Part model, mm, in its own coordinate system. Face numbers are marked on the shaded views. A direction names the side the tool comes from. Coordinates: 2 decimals unless noted, no trailing zeros. Loops run counter-clockwise (first coordinate to the right, second up) from the corner with the lowest first, then second, coordinate; pieces in that order, holes last. Notation, with made-up numbers: (31.25, 63) - (82.25, 63) arc R16 cw to (82.25, 68) - close; hole circle Ø3 at (-31, 20). An arc over 180 degrees is marked (long way). Use a Markdown table: item, result. Add a question column.
1) Band-saw the part on B-B (x = 0). Give the cut face in (y, z).
2) Probe probe 1 along X at (y, z) = (-3.25, -3); probe 2 along Y at (x, z) = (-6.5, 7); probe 3 along X at (y, z) = (8.5, -2). List the from-to ranges inside material, lowest first. Write a range as [from, to].
3) Band-saw the part on A-A (z = 0). Give the cut face in (x, y).
4) Pull direction Z, two halves, no side cores. Call the marked faces 3, 4 and 5: +Z half, -Z half, draft (parallel to the pull), parting line (faces both ways), or undercut.
5) Band-saw the part on C-C (y = -2). Give the cut face in (x, z).
6) Band-saw the part on D-D (y = 13). Give the cut face in (x, z).
7) Drop flat-ended pins along their axis: P1, Ø3, axis at y = 3.5, z = 6.5, coming from the -X side; P2, Ø4, axis at x = 13.5, y = 0.5, coming from the -Z side; P3, Ø6, axis at x = 11.5, z = 9, coming from the -Y side. Give the stop position or say it passes through.
8) Tool access for the marked faces 1 and 2: list every direction of +Z, -Z, +X, -X, +Y, -Y with a clear straight run to the whole face (end or side of a thin tool).
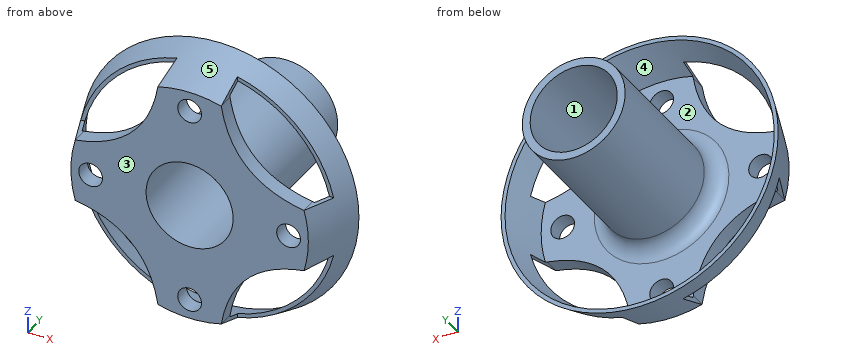
from build123d import *

# Parameters (mm, degrees)
SKETCH1_R           = 17.5
BOSS_EXTRUDE1_DEPTH = 7
BOSS_EXTRUDE1_DRAFT = -19.7
SKETCH5_R           = 17
CUT_EXTRUDE1_DEPTH  = 5
CUT_EXTRUDE1_DRAFT  = -19.7
CUT_EXTRUDE2_DEPTH  = 4
SKETCH7_R           = 5.5
CUT_EXTRUDE3_DEPTH  = 26.719642463
SKETCH8_R           = 1.5
CUT_EXTRUDE4_DEPTH  = 26.719642463
SKETCH9_R           = 6.5
BOSS_EXTRUDE2_DEPTH = 20
FILLET1_R           = 2
SKETCH10_R          = 5.5
CUT_EXTRUDE5_DEPTH  = 32.819805263


with BuildPart() as part:
    # Sketch1 → Boss-Extrude1 (with draft: the straight prism first)
    with BuildSketch(Plane(origin=(0, 0, 0), x_dir=(1, 0, 0), z_dir=(0, 1, 0))):
        Circle(SKETCH1_R)
    extrude(amount=-BOSS_EXTRUDE1_DEPTH)
    # Boss-Extrude1: the draft: its side faces are tilted about the plane it starts from
    boss_extrude1_sides = [part.faces().sort_by_distance(p)[0] for p in [
        (-17.5, -3.5, 0),
    ]]
    draft(boss_extrude1_sides, Plane(origin=(0, 0, 0), x_dir=(1, 0, 0), z_dir=(0, 1, 0)), BOSS_EXTRUDE1_DRAFT)


with BuildPart() as cut_extrude1_tool:
    # Sketch5 → Cut-Extrude1 (with draft: the straight prism first)
    with BuildSketch(Plane(origin=(0, 0, 0), x_dir=(1, 0, 0), z_dir=(0, 1, 0))):
        Circle(SKETCH5_R)
    extrude(amount=-CUT_EXTRUDE1_DEPTH)
    # Cut-Extrude1: the draft: its side faces are tilted about the plane it starts from
    cut_extrude1_sides = [cut_extrude1_tool.faces().sort_by_distance(p)[0] for p in [
        (-17, -2.5, 0),
    ]]
    draft(cut_extrude1_sides, Plane(origin=(0, 0, 0), x_dir=(1, 0, 0), z_dir=(0, 1, 0)), CUT_EXTRUDE1_DRAFT)


with BuildPart() as part_1:
    add(part.part)

    # Cut-Extrude1: cut by cut_extrude1_tool
    add(cut_extrude1_tool.part, mode=Mode.SUBTRACT)

    # Sketch6 → Cut-Extrude2 (cut)
    with BuildSketch(Plane.XZ.offset(7)):
        with BuildLine():
            add(Edge.make_bspline(
                [(-3.745787555, 17.094416503), (-3.800126667, 15.699556272), (-4, 14.450230262)],
                knots=[0, 0, 0, 0.108565408, 0.108565408, 0.108565408], degree=2))
            ThreePointArc((-3.745787555, 17.094416503), (-12.374368671, 12.374368671), (-17.094416503, 3.745787555))
            add(Edge.make_bspline(
                [(-14.450230262, 4), (-15.699556272, 3.800126667), (-17.094416503, 3.745787555)],
                knots=[0.891434592, 0.891434592, 0.891434592, 1, 1, 1], degree=2))
            ThreePointArc((-14.450230262, 4), (-10.602102495, 10.602102495), (-4, 14.450230262))
        make_face()
        with BuildLine():
            add(Edge.make_bspline(
                [(-4, 14.450230262), (-5.441294026, 5.441294026), (-14.450230262, 4)],
                knots=[0.108565408, 0.108565408, 0.108565408, 0.891434592, 0.891434592, 0.891434592], degree=2))
            ThreePointArc((-4, 14.450230262), (-10.602102495, 10.602102495), (-14.450230262, 4))
        make_face()
        with BuildLine():
            ThreePointArc((-17.094416503, -3.745787555), (-12.374368671, -12.374368671), (-3.745787555, -17.094416503))
            add(Edge.make_bspline(
                [(-3.745787555, -17.094416503), (-3.800126667, -15.699556272), (-4, -14.450230262)],
                knots=[0, 0, 0, 0.108565408, 0.108565408, 0.108565408], degree=2))
            ThreePointArc((-4, -14.450230262), (-10.602102495, -10.602102495), (-14.450230262, -4))
            add(Edge.make_bspline(
                [(-14.450230262, -4), (-15.699556272, -3.800126667), (-17.094416503, -3.745787555)],
                knots=[0.891434592, 0.891434592, 0.891434592, 1, 1, 1], degree=2))
        make_face()
        with BuildLine():
            ThreePointArc((-14.450230262, -4), (-10.602102495, -10.602102495), (-4, -14.450230262))
            add(Edge.make_bspline(
                [(-4, -14.450230262), (-5.441294026, -5.441294026), (-14.450230262, -4)],
                knots=[0.108565408, 0.108565408, 0.108565408, 0.891434592, 0.891434592, 0.891434592], degree=2))
        make_face()
        with BuildLine():
            ThreePointArc((4, -14.450230262), (10.602102495, -10.602102495), (14.450230262, -4))
            add(Edge.make_bspline(
                [(4, -14.450230262), (5.441294026, -5.441294026), (14.450230262, -4)],
                knots=[0.108565408, 0.108565408, 0.108565408, 0.891434592, 0.891434592, 0.891434592], degree=2))
        make_face()
        with BuildLine():
            ThreePointArc((3.745787555, -17.094416503), (12.374368671, -12.374368671), (17.094416503, -3.745787555))
            add(Edge.make_bspline(
                [(14.450230262, -4), (15.699556272, -3.800126667), (17.094416503, -3.745787555)],
                knots=[0.891434592, 0.891434592, 0.891434592, 1, 1, 1], degree=2))
            ThreePointArc((14.450230262, -4), (10.602102495, -10.602102495), (4, -14.450230262))
            add(Edge.make_bspline(
                [(3.745787555, -17.094416503), (3.800126667, -15.699556272), (4, -14.450230262)],
                knots=[0, 0, 0, 0.108565408, 0.108565408, 0.108565408], degree=2))
        make_face()
        with BuildLine():
            add(Edge.make_bspline(
                [(4, 14.450230262), (5.441294026, 5.441294026), (14.450230262, 4)],
                knots=[0.108565408, 0.108565408, 0.108565408, 0.891434592, 0.891434592, 0.891434592], degree=2))
            ThreePointArc((14.450230262, 4), (10.602102495, 10.602102495), (4, 14.450230262))
        make_face()
        with BuildLine():
            add(Edge.make_bspline(
                [(14.450230262, 4), (15.699556272, 3.800126667), (17.094416503, 3.745787555)],
                knots=[0.891434592, 0.891434592, 0.891434592, 1, 1, 1], degree=2))
            ThreePointArc((17.094416503, 3.745787555), (12.374368671, 12.374368671), (3.745787555, 17.094416503))
            add(Edge.make_bspline(
                [(3.745787555, 17.094416503), (3.800126667, 15.699556272), (4, 14.450230262)],
                knots=[0, 0, 0, 0.108565408, 0.108565408, 0.108565408], degree=2))
            ThreePointArc((4, 14.450230262), (10.602102495, 10.602102495), (14.450230262, 4))
        make_face()
    extrude(amount=-CUT_EXTRUDE2_DEPTH, mode=Mode.SUBTRACT)

    # Sketch7 → Cut-Extrude3 (cut, through all)
    with BuildSketch(Plane.XZ.offset(7)):
        with Locations(Location((0, 0, 0), (0, 0, 270))):
            Circle(SKETCH7_R)
    extrude(amount=-CUT_EXTRUDE3_DEPTH, mode=Mode.SUBTRACT)

    # Sketch8 → Cut-Extrude4 (cut, through all)
    with BuildSketch(Plane.XZ.offset(7)):
        with Locations(Location((-12.5, 0, 0), (0, 0, 270))):
            Circle(SKETCH8_R)
        with Locations(Location((0, 12.5, 0), (0, 0, 270))):
            Circle(SKETCH8_R)
        with Locations(Location((12.5, 0, 0), (0, 0, 270))):
            Circle(SKETCH8_R)
        with Locations(Location((0, -12.5, 0), (0, 0, 270))):
            Circle(SKETCH8_R)
    extrude(amount=-CUT_EXTRUDE4_DEPTH, mode=Mode.SUBTRACT)

    # Sketch9 → Boss-Extrude2 (add)
    with BuildSketch(Plane(origin=(0, -5, 0), x_dir=(1, 0, 0), z_dir=(0, 1, 0))):
        with Locations(Location((0, 0, 0), (0, 0, 270))):
            Circle(SKETCH9_R)
    extrude(amount=BOSS_EXTRUDE2_DEPTH)

    # Fillet1
    fillet1_edges = [part_1.edges().sort_by_distance(p)[0] for p in [
        (0, -5, -6.5),
    ]]
    fillet(fillet1_edges, radius=FILLET1_R)

    # Sketch10 → Cut-Extrude5 (cut, through all)
    with BuildSketch(Plane.XZ.offset(5)):
        with Locations(Location((0, 0, 0), (0, 0, 270))):
            Circle(SKETCH10_R)
    extrude(amount=-CUT_EXTRUDE5_DEPTH, mode=Mode.SUBTRACT)


solid = part_1.part
Answer block:
| question | item | result |
|---|---|---|
| 1 | outline | (-7, -14.99) - (0, -17.5) - (0, -17) - (-5, -15.21) - (-5, -14) - (-7, -14) - close; (-7, -11) - (-5, -11) - (-5, -8.5) arc R2 cw to (-3, -6.5) - (15, -6.5) - (15, -5.5) - (-7, -5.5) - close; (-7, 5.5) - (15, 5.5) - (15, 6.5) - (-3, 6.5) arc R2 cw to (-5, 8.5) - (-5, 11) - (-7, 11) - close; (-7, 14) - (-5, 14) - (-5, 15.21) - (0, 17) - (0, 17.5) - (-7, 14.99) - close |
| 2 | probe 1 | [-16.06, -15.55], [-5.78, -4.61], [4.61, 5.78], [15.55, 16.06] |
| 2 | probe 2 | [-7, -5] |
| 2 | probe 3 | [-6.18, -5.12], [5.12, 6.18] |
| 3 | outline | (-17.5, 0) - (-14.99, -7) - (-14, -7) - (-14, -5) - (-15.21, -5) - (-17, 0) - close; (-11, -7) - (-5.5, -7) - (-5.5, 15) - (-6.5, 15) - (-6.5, -3) arc R2 cw to (-8.5, -5) - (-11, -5) - close; (5.5, -7) - (11, -7) - (11, -5) - (8.5, -5) arc R2 cw to (6.5, -3) - (6.5, 15) - (5.5, 15) - close; (14, -7) - (14.99, -7) - (17.5, 0) - (17, 0) - (15.21, -5) - (14, -5) - close |
| 4 | face 3 | draft |
| 4 | face 4 | undercut |
| 4 | face 5 | parting line |
| 5 | outline | circle Ø33.57 at (0, 0); circle Ø13 at (0, 0); hole circle Ø32.57 at (0, 0); hole circle Ø11 at (0, 0) |
| 6 | outline | circle Ø13 at (0, 0); hole circle Ø11 at (0, 0) |
| 7 | P1 | x = -4.15 |
| 7 | P2 | z = -13.14 |
| 7 | P3 | y = -3 |
| 8 | face 1 | +Y, -Y |
| 8 | face 2 | +Y |
